Here's how the part is built. I have some questions about the finished solid (model axes, mm). A direction names the side the tool comes from. Round coordinates to 2 decimals unless told otherwise and drop trailing zeros. Write each loop counter-clockwise with the first axis right and the second up, starting at its lowest first coordinate (ties: lowest second). Pieces come first, ordered by that corner, then holes. Notation, with made-up numbers: (41.5, 22.25) -> (94.5, 22.25) arc R12 cw to (94.5, 40.25) -> close; hole circle Ø2 at (-5, -33). An arc over 180 degrees is marked (long way). Answer as CSV lines item,"result".
from build123d import *

# Parameters (mm, degrees)
SKETCH020_AS_DRAWN_W                      = 5
SKETCH020_AS_DRAWN_H                      = 5
EXTRUDE021_DEPTH                          = 25
EXTRUDE021_ONTO_SKETCH020_PLACEMENT_ANGLE = 30
SKETCH018_AS_DRAWN_W                      = 17.6
SKETCH018_AS_DRAWN_H                      = 20
SKETCH018_AS_DRAWN_W_2                    = 2.5
EXTRUDE019_DEPTH                          = 2
EXTRUDE019_ONTO_SKETCH018_PLACEMENT_ANGLE = 120
EXTRUDE018_DEPTH                          = 2.5
EXTRUDE018_ONTO_SKETCH017_PLACEMENT_ANGLE = 120
EXTRUDE017_DEPTH                          = 1.2
EXTRUDE016_DEPTH                          = 1.2
EXTRUDE014_DEPTH                          = 1
EXTRUDE015_DEPTH                          = 1
EXTRUDE015_ONTO_SKETCH015_PLACEMENT_ANGLE = 30
EXTRUDE013_DEPTH                          = 2
SKETCH019_AS_DRAWN_W                      = 3.5
SKETCH019_AS_DRAWN_H                      = 20
SKETCH019_AS_DRAWN_W_2                    = 7.5
SKETCH019_AS_DRAWN_W_3                    = 20.1
EXTRUDE020_DEPTH                          = 2
EXTRUDE020_ONTO_SKETCH019_PLACEMENT_ANGLE = 120


with BuildPart() as extrude021:
    # Sketch020 as drawn → Extrude021 (new)
    with BuildSketch(Plane.XY):
        with BuildLine():
            ThreePointArc((-17.5, 26.7697348593), (-19.5, 24.7697348593), (-17.5, 22.7697348593))
            Line((-17.5, 22.7697348593), (1, 22.7697348593))
            ThreePointArc((1, 22.7697348593), (3, 24.7697348593), (1, 26.7697348593))
            Line((1, 26.7697348593), (-17.5, 26.7697348593))
        make_face()
        with BuildLine():
            ThreePointArc((-31.5, 22.7697348593), (-29.5, 24.7697348593), (-31.5, 26.7697348593))
            Line((-31.5, 26.7697348593), (-37.5, 26.7697348593))
            ThreePointArc((-37.5, 26.7697348593), (-39.5, 24.7697348593), (-37.5, 22.7697348593))
            Line((-37.5, 22.7697348593), (-31.5, 22.7697348593))
        make_face()
        with BuildLine():
            ThreePointArc((14.5, 26.7697348593), (12.5, 24.7697348593), (14.5, 22.7697348593))
            Line((14.5, 22.7697348593), (20.5, 22.7697348593))
            ThreePointArc((20.5, 22.7697348593), (22.5, 24.7697348593), (20.5, 26.7697348593))
            Line((20.5, 26.7697348593), (14.5, 26.7697348593))
        make_face()
        with Locations((31, 27.0697348593)):
            Rectangle(SKETCH020_AS_DRAWN_W, SKETCH020_AS_DRAWN_H)
        with Locations((38.5, 27.0697348593)):
            Rectangle(SKETCH020_AS_DRAWN_W, SKETCH020_AS_DRAWN_H)
    extrude(amount=-EXTRUDE021_DEPTH)


with BuildPart() as extrude021_1:
    # Extrude021 onto Sketch020 placement: moved
    add(extrude021.part.moved(Location((0, -21.15, 36.6328745801))).rotate(Axis((0, -21.15, 36.6328745801), (1, 0, 0)), EXTRUDE021_ONTO_SKETCH020_PLACEMENT_ANGLE))


with BuildPart() as extrude019:
    # Sketch018 as drawn → Extrude019 (new)
    with BuildSketch(Plane.XY):
        with Locations((34.8, 30.3)):
            Rectangle(SKETCH018_AS_DRAWN_W, SKETCH018_AS_DRAWN_H)
        with Locations((-24.25, 30.3)):
            Rectangle(SKETCH018_AS_DRAWN_W_2, SKETCH018_AS_DRAWN_H)
        with Locations((7.75, 30.3)):
            Rectangle(SKETCH018_AS_DRAWN_W_2, SKETCH018_AS_DRAWN_H)
    extrude(amount=EXTRUDE019_DEPTH)


with BuildPart() as extrude019_1:
    # Extrude019 onto Sketch018 placement: moved
    add(extrude019.part.moved(Location((0, 23.4430780618, 13.5348674296))).rotate(Axis((0, 23.4430780618, 13.5348674296), (1, 0, 0)), EXTRUDE019_ONTO_SKETCH018_PLACEMENT_ANGLE))


with BuildPart() as extrude018:
    # Sketch017 as drawn → Extrude018 (new)
    with BuildSketch(Plane.XY):
        Polygon((-43.5, 40.3), (43.6, 40.3), (43.6, 20.3), (23.5, 20.3), (23.5, 40.2), (11.5, 40.2), (11.5, 20.3), (4, 20.3), (4, 37.8), (-20.5, 37.8), (-20.5, 20.3), (-29, 20.3), (-29, 37.8), (-40, 37.8), (-40, 20.3), (-43.5, 20.3), align=None)
    extrude(amount=EXTRUDE018_DEPTH)


with BuildPart() as extrude018_1:
    # Extrude018 onto Sketch017 placement: moved
    add(extrude018.part.moved(Location((0, 25.6081415713, 14.7848674296))).rotate(Axis((0, 25.6081415713, 14.7848674296), (1, 0, 0)), EXTRUDE018_ONTO_SKETCH017_PLACEMENT_ANGLE))


with BuildPart() as extrude017:
    # Sketch016 → Extrude017 (new body)
    with BuildSketch(Plane.YZ):
        with BuildLine():
            Line((5.4581415713, 49.6856912021), (-16.1924935233, 37.1856912021))
            ThreePointArc((-16.1924935233, 37.1856912021), (-1.0123345563, 25.5375455449), (17.9581415713, 28.0350561075))
            Line((5.4581415713, 49.6856912021), (17.9581415713, 28.0350561075))
        make_face()
    extrude(amount=EXTRUDE017_DEPTH)


with BuildPart() as extrude017_1:
    # Extrude017 placement: moved
    add(extrude017.part.moved(Location((-44.7, 0, 0))))


with BuildPart() as extrude016:
    # Sketch016 → Extrude016 (new body)
    with BuildSketch(Plane.YZ):
        with BuildLine():
            Line((5.4581415713, 49.6856912021), (-16.1924935233, 37.1856912021))
            ThreePointArc((-16.1924935233, 37.1856912021), (-1.0123345563, 25.5375455449), (17.9581415713, 28.0350561075))
            Line((5.4581415713, 49.6856912021), (17.9581415713, 28.0350561075))
        make_face()
    extrude(amount=EXTRUDE016_DEPTH)


with BuildPart() as extrude016_1:
    # Extrude016 placement: moved
    add(extrude016.part.moved(Location((43.6, 0, 0))))


with BuildPart() as extrude014:
    # Facebinder001 → Extrude014 (new body)
    with BuildSketch(Plane(origin=(0, -11.8962827712, 40.8208101747), x_dir=(-1, 0, 0), z_dir=(0, -0.5, 0.8660254038))):
        with BuildLine():
            Line((44.85, -21.4618128624), (44.85, 15.708219608))
            add(Edge.make_bspline(
                [(44.85, 15.708219608), (44.85, 21.5971923538), (39.75, 21.5971923538)],
                knots=[4.7123889804, 4.7123889804, 4.7123889804, 6.2831853072, 6.2831853072, 6.2831853072], degree=2, weights=[1, 0.7071067812, 1]))
            Line((39.75, 21.5971923538), (-39.75, 21.5971923538))
            add(Edge.make_bspline(
                [(-39.75, 21.5971923538), (-44.85, 21.5971923538), (-44.85, 15.708219608)],
                knots=[0, 0, 0, 1.5707963268, 1.5707963268, 1.5707963268], degree=2, weights=[1, 0.7071067812, 1]))
            Line((-44.85, 15.708219608), (-44.85, -21.4618128624))
            Line((-44.85, -21.4618128624), (44.85, -21.4618128624))
        make_face()
    extrude(amount=-EXTRUDE014_DEPTH)


with BuildPart() as extrude015:
    # Sketch015 as drawn → Extrude015 (new)
    with BuildSketch(Plane.XY):
        with BuildLine():
            Line((-47.25, -5.6002976111), (-47.25, 31.8410161514))
            Line((-47.25, 31.8410161514), (-47.25, 33.8410161514))
            Line((-47.25, 33.8410161514), (-45.25, 33.8410161514))
            Line((-45.25, 33.8410161514), (45.25, 33.8410161514))
            Line((45.25, 33.8410161514), (47.25, 33.8410161514))
            Line((47.25, 33.8410161514), (47.25, 31.8410161514))
            Line((47.25, 31.8410161514), (47.25, -5.6002976111))
            add(Edge.make_bspline(
                [(39.75, -14.260551649), (47.25, -14.260551649), (47.25, -5.6002976111)],
                knots=[0, 0, 0, 1.5707963268, 1.5707963268, 1.5707963268], degree=2, weights=[1, 0.7071067812, 1]))
            Line((39.75, -14.260551649), (-39.75, -14.260551649))
            add(Edge.make_bspline(
                [(-47.25, -5.6002976111), (-47.25, -14.260551649), (-39.75, -14.260551649)],
                knots=[4.7123889804, 4.7123889804, 4.7123889804, 6.2831853072, 6.2831853072, 6.2831853072], degree=2, weights=[1, 0.7071067812, 1]))
        make_face()
    extrude(amount=EXTRUDE015_DEPTH)


with BuildPart() as extrude015_1:
    # Extrude015 onto Sketch015 placement: moved
    add(extrude015.part.moved(Location((0, -20.65, 35.7668491763))).rotate(Axis((0, -20.65, 35.7668491763), (1, 0, 0)), EXTRUDE015_ONTO_SKETCH015_PLACEMENT_ANGLE))


with BuildPart() as inner_complete:
    # Facebinder → Extrude013 (new body)
    with BuildSketch(Plane(origin=(0, 18.5885038732, 30.9432365735), x_dir=(1, 0, 0), z_dir=(0, 0.8660254038, 0.5))):
        with BuildLine():
            Line((39.75, 24.0229922536), (-39.75, 24.0229922536))
            add(Edge.make_bspline(
                [(-39.75, 24.0229922536), (-44.85, 24.0229922536), (-44.85, 13.8229922536)],
                knots=[0, 0, 0, 1.5707963268, 1.5707963268, 1.5707963268], degree=2, weights=[1, 0.7071067812, 1]))
            Line((-44.85, 13.8229922536), (-44.85, -23.7966229887))
            Line((-44.85, -23.7966229887), (44.85, -23.7966229887))
            Line((44.85, -23.7966229887), (44.85, 13.8229922536))
            add(Edge.make_bspline(
                [(44.85, 13.8229922536), (44.85, 24.0229922536), (39.75, 24.0229922536)],
                knots=[4.7123889804, 4.7123889804, 4.7123889804, 6.2831853072, 6.2831853072, 6.2831853072], degree=2, weights=[1, 0.7071067812, 1]))
        make_face()
    extrude(amount=-EXTRUDE013_DEPTH)

    # Connect003: union Extrude014, Extrude015
    add(extrude014.part)
    add(extrude015_1.part)


with BuildPart() as cut006:
    # Sketch019 as drawn → Extrude020 (new)
    with BuildSketch(Plane.XY):
        with Locations((-41.75, 30.3)):
            Rectangle(SKETCH019_AS_DRAWN_W, SKETCH019_AS_DRAWN_H)
        Polygon((-29, 40.3), (-20.5, 40.3), (-20.5, 20.3), (-25.5, 20.3), (-25.5, 35.3), (-29, 35.3), align=None)
        with Locations((7.75, 30.3)):
            Rectangle(SKETCH019_AS_DRAWN_W_2, SKETCH019_AS_DRAWN_H)
        with Locations((33.55, 30.3)):
            Rectangle(SKETCH019_AS_DRAWN_W_3, SKETCH019_AS_DRAWN_H)
    extrude(amount=EXTRUDE020_DEPTH)


with BuildPart() as cut006_1:
    # Extrude020 onto Sketch019 placement: moved
    add(cut006.part.moved(Location((0, 21.7110272543, 12.5348674296))).rotate(Axis((0, 21.7110272543, 12.5348674296), (1, 0, 0)), EXTRUDE020_ONTO_SKETCH019_PLACEMENT_ANGLE))

    # Connect004: union Extrude019, Extrude018, Extrude017, Extrude016, inner_complete
    add(extrude019_1.part)
    add(extrude018_1.part)
    add(extrude017_1.part)
    add(extrude016_1.part)
    add(inner_complete.part)

    # Cut006: cut Extrude021
    add(extrude021_1.part, mode=Mode.SUBTRACT)


solid = cut006_1.part
Item 1: Suppose I cut it at A-A, the plane x = -35. List the corners of the cut face in (y, z) for me.
Results found:
outline,"(-33.5, 29.5) -> (-33, 28.64) -> (-30.6, 30.02) -> (-30.1, 29.16) -> (-0.43, 46.29) -> (-1.43, 48.02) -> close; (2.03, 50.02) -> (3.03, 48.29) -> (3.29, 48.44) -> (4.54, 46.27) -> (6.71, 47.52) -> (28.87, 9.14) -> (30.6, 10.14) -> (6.69, 51.55) -> (8.66, 52.69) -> (8.16, 53.55) -> close"
Item 2: Suppose I cut it at B-B, the plane x = 35. List the corners of the cut face in (y, z) for me.
Results found:
outline,"(-33.5, 29.5) -> (-33, 28.64) -> (-30.6, 30.02) -> (-30.1, 29.16) -> (-0.17, 46.44) -> (9.83, 29.12) -> (15.46, 32.37) -> (28.87, 9.14) -> (30.6, 10.14) -> (6.69, 51.55) -> (8.66, 52.69) -> (8.16, 53.55) -> close"
Item 3: I need wall thicknesses on L1, parallel to Y at x = -10.5, z = 47; L2, parallel to Z at x = 11, y = 5; L3, parallel to Z at x = -42, y = 8. Which ranges of each line are inside material? Lowest first, please.
Results found:
L1,"y = -3.19 to -0.84, 4.12 to 5.81, 7.01 to 9.32"
L2,"z = 37.48 to 41.48, 45.48 to 51.73"
L3,"z = 32.28 to 36.28, 40.28 to 49.28, 52.31 to 53.46"
Item 4: Will these pins go through, and if not, where does the flat tip stop? pin 1 (6 mm diameter, centred on x = 4.5, y = -6.5, fed in from +Z); pin 2 (12.5 mm diameter, centred on y = -1.5, z = 32, fed in from -X); pin 3 (9.5 mm diameter, centred on y = 8, z = 43, fed in from +X).
Results found:
pin 1,"stops at z = 46.82"
pin 2,"stops at x = -44.7"
pin 3,"stops at x = 44.85"
Item 5: If we mould it in two halves opening along Z, with no side actions, what happens to faces 1 (the flat face through (7.8, 12.68, 30.76)), 2 (the flat face through (28.5, 8, 41)), 3 (the flat face through (4, 10, 39))? For each: pulls with the +Z half, pulls with the -Z half, needs draft (parallel to the pull), parting line crosses it, or undercut.
Results found:
face 1,"pulls with the -Z half"
face 2,"undercut"
face 3,"needs draft"
Item 6: Suppose I cut it at D-D, the plane x = 16. List the corners of the cut face in (y, z) for me.
Results found:
outline,"(-33.5, 29.5) -> (-33, 28.64) -> (-30.6, 30.02) -> (-30.1, 29.16) -> (-0.43, 46.29) -> (-1.43, 48.02) -> close; (2.03, 50.02) -> (3.03, 48.29) -> (3.29, 48.44) -> (3.34, 48.35) -> (5.51, 49.6) -> (28.87, 9.14) -> (30.6, 10.14) -> (6.69, 51.55) -> (8.66, 52.69) -> (8.16, 53.55) -> close"
Item 7: For faces 4 (the flat face through (-44.85, 12, 39)), 5 (the flat face through (24.73, 6.49, 38.9)), 6 (the flat face through (-29, 2, 45)), which set-ups out of +Z, -Z, +X, -X, +Y, -Y let a thin tool reach every point of the face, with its end or its side?
Results found:
face 4,"-Z, -X, +Y"
face 5,"none"
face 6,"-Z"
Item 8: Suppose I cut it at C-C, the plane y = -5. List the corners of the cut face in (x, z) for me, then the cut area to 3 significant figures.
Results found:
outline,"(-47.25, 44.8) -> (-44.85, 44.8) -> (-44.85, 43.65) -> (-44.7, 43.65) -> (-44.7, 26.98) -> (-43.5, 26.98) -> (-43.5, 43.65) -> (43.6, 43.65) -> (43.6, 26.98) -> (44.8, 26.98) -> (44.8, 43.65) -> (44.85, 43.65) -> (44.85, 44.8) -> (47.25, 44.8) -> (47.25, 45.96) -> (-47.25, 45.96) -> close"
area,"253 mm²"
